For this review, use the dimensioned drawing (mm, ordinates from the lowest corner) and the shaded views. A direction names the side the tool comes from. Round coordinates to 2 decimals unless told otherwise and drop trailing zeros. Write each loop counter-clockwise with the first axis right and the second up, starting at its lowest first coordinate (ties: lowest second). Pieces come first, ordered by that corner, then holes. Notation, with made-up numbers: M 15,71 L 52,71 A18 cw 52,103 Z; hole C 88.25,22.25 d9. An arc over 180 degrees is marked long. One line per question, with ' | ' between items.
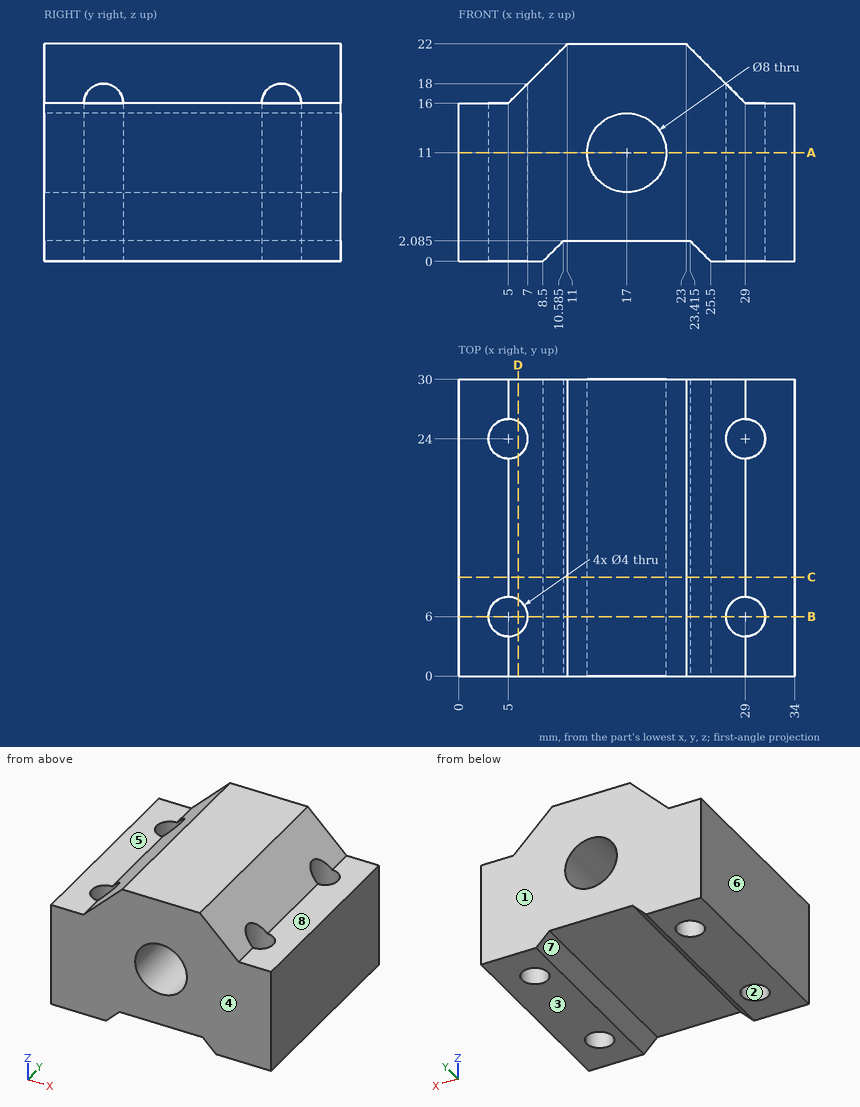
Item 1: Take a section at A-A (z = 11). Write out the cut boundary in (x, y).
Results:
outline: M 0,0 L 13,0 L 13,30 L 0,30 Z; M 21,0 L 34,0 L 34,30 L 21,30 Z; hole C 5,6 d4; hole C 5,24 d4; hole C 29,6 d4; hole C 29,24 d4
Item 2: Insertion check: pin 1 Ø3.5 at (x, y) = (5, 24) entering from +Z; pin 2 Ø2.5 at (x, y) = (2, 17) entering from +Z; pin 3 Ø6.5 at (x, y) = (29, 6) entering from +Z; pin 4 Ø10 at (x, y) = (28.5, 3) entering from +Z. Each pin has a flat end and moves straight along its axis. Give the tip position at first contact, or say it passes through.
Results:
pin 1: through | pin 2: z = 16 | pin 3: z = 19.25 | pin 4: z = 21.5
Item 3: Take a section at B-B (y = 6). Write out the cut boundary in (x, z) (3 decimals), then the cut area to 3 significant figures.
Results:
outline: M 0,0 L 3,0 L 3,16 L 0,16 Z; M 7,0 L 8.5,0 L 10.585,2.085 L 23.415,2.085 L 25.5,0 L 27,0 L 27,18 L 23,22 L 11,22 L 7,18 Z; M 31,0 L 34,0 L 34,16 L 31,16 Z; hole C 17,11 d8 | area: 439 mm2
Item 4: Take a section at C-C (y = 10). Write out the cut boundary in (x, z) (3 decimals).
Results:
outline: M 0,0 L 8.5,0 L 10.585,2.085 L 23.415,2.085 L 25.5,0 L 34,0 L 34,16 L 29,16 L 23,22 L 11,22 L 5,16 L 0,16 Z; hole C 17,11 d8
Item 5: Take a section at D-D (x = 6). Write out the cut boundary in (y, z), then the cut area to 3 significant figures.
Results:
outline: M 0,0 L 4.27,0 L 4.27,17 L 0,17 Z; M 7.73,0 L 22.27,0 L 22.27,17 L 7.73,17 Z; M 25.73,0 L 30,0 L 30,17 L 25.73,17 Z | area: 392 mm2
Item 6: Mouldability with a two-part tool opening along Y and no side actions: class the marked faces 1, 2, 3 and 4 as +Y half, -Y half, draft (parallel to the pull), parting line (faces both ways), or undercut.
Results:
face 1: +Y half | face 2: undercut | face 3: draft | face 4: -Y half
Item 7: Machinability: for the marked faces 5, 6, 7 and 8, which of the approach directions +Z, -Z, +X, -X, +Y, -Y give a long, thin tool a straight path to every point of the face, cutting with its end or side? Answer none if there is none.
Results:
face 5: +Z, -X, +Y, -Y | face 6: +Z, -Z, -X, +Y, -Y | face 7: -Z, +Y, -Y | face 8: +Z, +X, +Y, -Y
Item 8: To check wall thickness, follow line 1 along X through (y, z) = (24, 6); line 2 along Y through (x, z) = (5, 2.5); line 3 along Y through (x, z) = (6, 11.5). State the ranges of each line that lie inside material, in increasing order. Write a range as from..to.
Results:
line 1: 0..3, 7..27, 31..34 | line 2: 0..4, 8..22, 26..30 | line 3: 0..4.27, 7.73..22.27, 25.73..30
